```python
from build123d import *

# Parameters (mm, degrees)
SKETCH1_W               = 25.4
SKETCH1_H               = 10.16
REVOLVE1_ANGLE          = 180
SKETCH4_W               = 6.29000012
SKETCH4_H               = 3.69
SKETCH6_W               = 3.294985449
SKETCH6_H               = 5.974962046
BOSS_EXTRUDE1_DEPTH     = 5.08
SKETCH7_R               = 3.22
BOSS_EXTRUDE7_DEPTH     = 12.7
SKETCH9_W               = 3.294985449
SKETCH9_H               = 5.974962046
BOSS_EXTRUDE8_DEPTH     = 3.302
CUT_EXTRUDE1_DEPTH      = 3.302
CUT_EXTRUDE1_DEPTH_BACK = 3.302
SKETCH11_R              = 2.375
CUT_EXTRUDE2_DEPTH      = 2.54
CUT_EXTRUDE2_DEPTH_BACK = 12.446
BOSS_EXTRUDE11_DEPTH    = 3.81
SKETCH14_R              = 2.420907349
CUT_EXTRUDE3_DEPTH      = 22.606


with BuildPart() as part:
    # Sketch1 → Revolve1 (revolve)
    with BuildSketch(Plane(origin=(0, 0, 0), x_dir=(1, 0, 0), z_dir=(0, 1, 0))):
        with Locations((12.7, 5.451011236)):
            Rectangle(SKETCH1_W, SKETCH1_H)
    revolve(axis=Axis((0, 0, -0.371011236), (1, 0, 0)), revolution_arc=REVOLVE1_ANGLE)

    # Sweep1: sweep along a path in Sketch5
    with BuildLine(Plane.XY) as sweep1_path:
        ThreePointArc((12.7, 0), (20.315428689, -15.331843414), (12.392600359, -30.5071183))
    # Sketch4 → Sweep1 (sweep)
    with BuildSketch(Plane(origin=(0, 0, 0), x_dir=(1, 0, 0), z_dir=(0, 1, 0))):
        with Locations((12.7, 0.371011236)):
            Rectangle(SKETCH4_W, SKETCH4_H)
    sweep(path=sweep1_path.line)

    # Sketch6 → Boss-Extrude1 (add)
    with BuildSketch(Plane(origin=(20.164340987, -6.538110874, 0), x_dir=(0, 0, 1), z_dir=(-0.95124601, 0.308433183, 0))):
        with Locations((-0.361104817, -25.204906835)):
            Rectangle(SKETCH6_W, SKETCH6_H)
    extrude(amount=BOSS_EXTRUDE1_DEPTH)

    # Sketch7 → Boss-Extrude7 (add)
    with BuildSketch(Plane(origin=(15.332011256, -4.971270302, 0), x_dir=(0, 0, 1), z_dir=(-0.95124601, 0.308433183, 0))):
        with Locations((-0.361104816, -31.160979548)):
            Circle(SKETCH7_R)
    extrude(amount=-BOSS_EXTRUDE7_DEPTH)

    # Sketch9 → Boss-Extrude8 (add)
    with BuildSketch(Plane(origin=(15.332011256, -4.971270302, 0), x_dir=(0, 0, 1), z_dir=(-0.95124601, 0.308433183, 0))):
        with Locations((-0.361104817, -25.204906835)):
            Rectangle(SKETCH9_W, SKETCH9_H)
    extrude(amount=BOSS_EXTRUDE8_DEPTH)

    # Sketch10 → Cut-Extrude1 (cut, two sides)
    with BuildSketch(Plane.XY) as cut_extrude1_sk:
        with BuildLine():
            Line((3.495528998, -30.770720391), (5.338405562, -25.087061585))
            Line((5.338405562, -25.087061585), (13.311749617, -27.672348528))
            add(Edge.make_bspline(
                [(13.311749617, -27.672348528), (8.683653097, -30.129373505), (3.495528998, -30.770720391)],
                knots=[0, 0, 0, 1, 1, 1], degree=2))
        make_face()
    extrude(amount=CUT_EXTRUDE1_DEPTH, mode=Mode.SUBTRACT)
    extrude(cut_extrude1_sk.sketch, amount=-CUT_EXTRUDE1_DEPTH_BACK, mode=Mode.SUBTRACT)

    # Sketch11 → Cut-Extrude2 (cut, two sides)
    with BuildSketch(Plane(origin=(27.412835582, -8.888371731, 0), x_dir=(0, 0, -1), z_dir=(0.95124601, -0.308433183, 0))) as cut_extrude2_sk:
        with Locations((0.39169909, -31.12675273)):
            Circle(SKETCH11_R)
    extrude(amount=CUT_EXTRUDE2_DEPTH, mode=Mode.SUBTRACT)
    extrude(cut_extrude2_sk.sketch, amount=-CUT_EXTRUDE2_DEPTH_BACK, mode=Mode.SUBTRACT)

    # Sketch13 → Boss-Extrude11 (add)
    with BuildSketch(Plane(origin=(27.412835582, -8.888371731, 0), x_dir=(0, 0, -1), z_dir=(0.95124601, -0.308433183, 0))):
        Polygon((-2.207938212, -40.151875097), (-0.189276492, -34.333593678), (-2.341873796, -32.910924296), (-4.569820403, -39.332416424), (-4.097443964, -39.496308159), (-3.315450943, -37.242411221), (-1.898321628, -37.734086425), (-2.68031465, -39.987983362), align=None)
        with BuildLine():
            Line((-3.374575741, -43.514412461), (-2.207938212, -40.151875097))
            Line((-2.207938212, -40.151875097), (-2.68031465, -39.987983362))
            Line((-2.68031465, -39.987983362), (-3.462307672, -42.241880299))
            ThreePointArc((-3.462307672, -42.241880299), (-3.5785484, -42.37264764), (-3.75320948, -42.382919506))
            Line((-3.75320948, -42.382919506), (-4.73839778, -42.041106905))
            ThreePointArc((-4.73839778, -42.041106905), (-4.86916512, -41.924866176), (-4.879436986, -41.750205096))
            Line((-4.879436986, -41.750205096), (-4.097443964, -39.496308159))
            Line((-4.097443964, -39.496308159), (-4.569820403, -39.332416424))
            Line((-4.569820403, -39.332416424), (-5.736457932, -42.694953789))
            ThreePointArc((-5.736457932, -42.694953789), (-5.726186066, -42.869614869), (-5.595418726, -42.985855597))
            Line((-5.595418726, -42.985855597), (-3.66547755, -43.655451668))
            ThreePointArc((-3.66547755, -43.655451668), (-3.490816469, -43.645179802), (-3.374575741, -43.514412461))
        make_face()
    extrude(amount=-BOSS_EXTRUDE11_DEPTH)

    # Sketch14 → Cut-Extrude3 (cut)
    with BuildSketch(Plane(origin=(27.412835582, -8.888371731, 0), x_dir=(0, 0, -1), z_dir=(0.95124601, -0.308433183, 0))):
        with Locations((0.361104816, -31.160979548)):
            Circle(SKETCH14_R)
    extrude(amount=-CUT_EXTRUDE3_DEPTH, mode=Mode.SUBTRACT)


solid = part.part
```
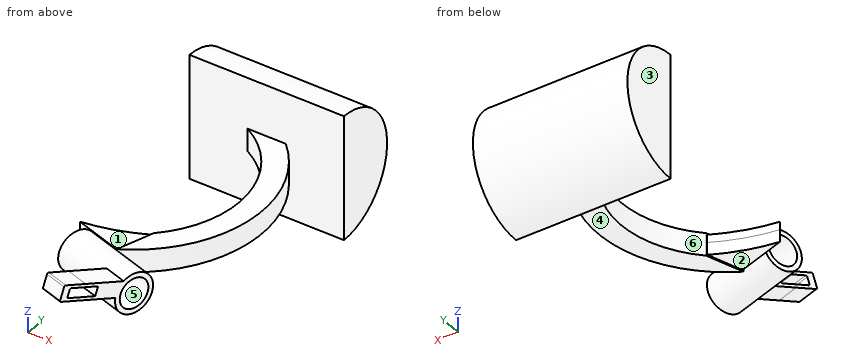
For this review, take the finished solid that the model builds, in its own axes (mm). Face numbers are marked on the shaded views. A direction names the side the tool comes from. Coordinates: 2 decimals unless noted, no trailing zeros. Loops run counter-clockwise (first coordinate to the right, second up) from the corner with the lowest first, then second, coordinate; pieces in that order, holes last.
1. Add section A-A, the plane x = 8. Count the separate pieces of the cut face and the enclosed holes in it, then the cut area to 3 significant figures.
2. Mouldability with a two-part tool opening along Z and no side actions: class the marked faces 4, 5 and 6 as +Z half, -Z half, draft (parallel to the pull), parting line (faces both ways), or undercut.
3. Add section C-C, the plane z = -4.75. Give the boundary of the cut face in (x, y), then the cut area to 3 significant figures.
4. Insertion check: P1, Ø5, axis at x = 19, y = -38, coming from the +Z side; P2, Ø3, axis at x = 8.5, z = 2, coming from the -Y side; P3, Ø6.5, axis at x = 10.5, y = -29.5, coming from the +Z side. Each pin has a flat end and moves straight along its axis. Give the tip position at first contact, or say it passes through.
5. For line 1 (Y direction, x = 11.5, z = 0.75); line 2 (Z direction, x = 9.75, y = -37.5); line 3 (Z direction, x = 16, y = -1.5), list the stretches that pass through material, from the lowest coordinate up.
6. For the marked faces 1, 2 and 3, list the 3-axis set-ups (+Z, -Z, +X, -X, +Y, -Y) from which the entire face can be reached by the end or side of a thin tool; tool diameter is ignored.
7. Add section B-B, the plane x = 23. Give the boundary of the cut face in (y, z).
8. Add section D-D, the plane z = -9. Give the boundary of the cut face in (x, y), then the cut area to 3 significant figures.
Result:
1. separate pieces: 2
1. enclosed holes: 1
1. area: 184 mm2
2. face 4: -Z half
2. face 5: undercut
2. face 6: draft
3. outline: (0, 0) - (25.4, 0) - (25.4, 9.17) - (0, 9.17) - close
3. area: 233 mm2
4. P1: stops at z = 2.86
4. P2: stops at y = -38.96
4. P3: stops at z = 1.47
5. line 1: y = -39.66 to -38.75, -34.23 to -28.56, -1.21 to 10.1
5. line 2: z = -3.21 to -2.26, 1.54 to 2.49
5. line 3: z = -2.22 to 1.47
6. face 1: +Z
6. face 2: -Z
6. face 3: +Z, -Z, -X, +Y, -Y
7. outline: (0, -10.53) arc R10.16 ccw to (0, 9.79) - close
8. outline: (0, 0) - (25.4, 0) - (25.4, 5.36) - (0, 5.36) - close
8. area: 136 mm2
